Input: part model. Units: mm. Frame: model coordinates. Coordinates: 2 decimals unless noted, no trailing zeros. Write each loop counter-clockwise with the first axis right and the second up, starting at its lowest first coordinate (ties: lowest second). Pieces come first, ordered by that corner, then holes. Notation, with made-up numbers: M -21.75,72 L 4.25,72 A34 cw 4.25,103 Z; hole C 46.25,-27 d8. An arc over 180 degrees is marked long. Write each question's results on one line, items separated by ' | '. Start each with the question number.
1. Section query B-B, the plane z = 0. Output: boundary loops of the cut face in (x, y).
2. Ray query, probe 1 along X at (y, z) = (-1.15, 0); probe 2 along Y at (x, z) = (3.25, 5); probe 3 along X at (y, z) = (-0.8, 0). Return the intervals inside material, ascending.
3. Section query A-A, the plane x = 0. Output: boundary loops of the cut face in (y, z).
```python
from build123d import *

# Parameters (mm, degrees)
CROQUIS1_R            = 5.5
CORTAR_EXTRUIR1_DEPTH = 10


with BuildPart() as part:
    # Croquis2 → Revolución1 (revolve)
    with BuildSketch(Plane.XY):
        Polygon((0, 0), (6, 0), (6, -0.5), (5.75, -0.5), (5.75, -1), (6, -1), (6, -1.5), (0, -1.5), align=None)
    revolve(axis=Axis((0, -1.5, 0), (0, 1, 0)))

    # Croquis1 → Cortar-Extruir1 (cut)
    with BuildSketch(Plane(origin=(0, 0, 0), x_dir=(1, 0, 0), z_dir=(0, 1, 0))):
        with Locations(Location((0, 0, 0), (0, 0, 270))):
            Circle(CROQUIS1_R)
    extrude(amount=-CORTAR_EXTRUIR1_DEPTH, mode=Mode.SUBTRACT)


solid = part.part
```
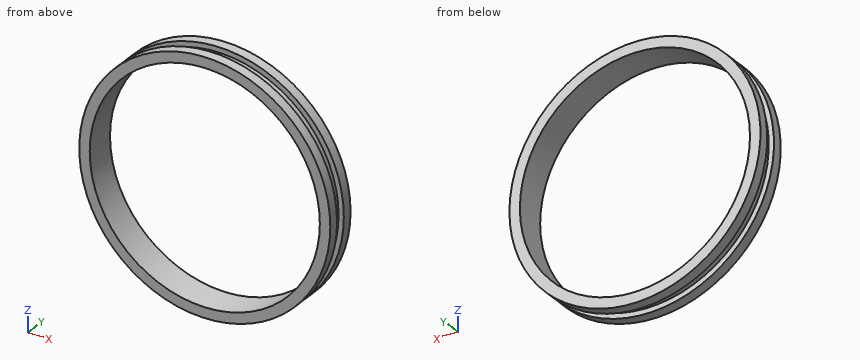
Answer:
1) outline: M -6,-1.5 L -5.5,-1.5 L -5.5,0 L -6,0 L -6,-0.5 L -5.75,-0.5 L -5.75,-1 L -6,-1 Z; M 5.5,-1.5 L 6,-1.5 L 6,-1 L 5.75,-1 L 5.75,-0.5 L 6,-0.5 L 6,0 L 5.5,0 Z
2) probe 1: -6 to -5.5, 5.5 to 6 | probe 2: -1.5 to -1, -0.5 to 0 | probe 3: -5.75 to -5.5, 5.5 to 5.75
3) outline: M -1.5,-6 L -1,-6 L -1,-5.75 L -0.5,-5.75 L -0.5,-6 L 0,-6 L 0,-5.5 L -1.5,-5.5 Z; M -1.5,5.5 L 0,5.5 L 0,6 L -0.5,6 L -0.5,5.75 L -1,5.75 L -1,6 L -1.5,6 Z
